Read the model definition and answer for the solid it produces. Units are mm, in the model's axes. Face numbers are marked on the shaded views. A direction names the side the tool comes from. Coordinates: 2 decimals unless noted, no trailing zeros. Order: outer loops, then holes, each group sorted by start corner. A loop starts at its lowest first (then second) coordinate and runs counter-clockwise, first axis right, second up. Notation, with made-up numbers: M 14,-8.5 L 56,-8.5 A9 cw 56,4.5 Z; hole C -22,74.25 d4. An arc over 180 degrees is marked long. Put each result on its own line as item: value.
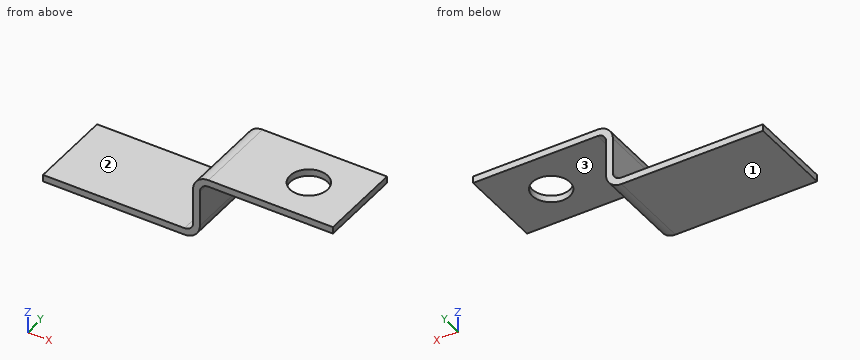
from build123d import *

# Parameters (mm, degrees)
SKETCH1_W           = 34
SKETCH1_H           = 10
BOSS_EXTRUDE1_DEPTH = 7.8
SKETCH2_W           = 15.6
SKETCH2_H           = 7
CUT_EXTRUDE1_DEPTH  = 63.432123894
SKETCH3_W           = 17.6
SKETCH3_H           = 7
CUT_EXTRUDE2_DEPTH  = 63.432123894
HOLE1_D             = 4.4
HOLE1_DEPTH         = 7.8
FILLET1_R           = 1
FILLET2_R           = 1
FILLET3_R           = 1.8
FILLET4_R           = 1.8


with BuildPart() as part:
    # Sketch1 → Boss-Extrude1 (new body)
    with BuildSketch(Plane.XY.offset(4.484761641)):
        with Locations((-44.46264725, 0)):
            Rectangle(SKETCH1_W, SKETCH1_H)
    extrude(amount=-BOSS_EXTRUDE1_DEPTH)

    # Sketch2 → Cut-Extrude1 (cut, through all)
    with BuildSketch(Plane(origin=(0, 5, 0), x_dir=(-1, 0, 0), z_dir=(0, 1, 0))):
        with Locations((35.26264725, 0.184761641)):
            Rectangle(SKETCH2_W, SKETCH2_H)
    extrude(amount=-CUT_EXTRUDE1_DEPTH, mode=Mode.SUBTRACT)

    # Sketch3 → Cut-Extrude2 (cut, through all)
    with BuildSketch(Plane(origin=(0, 5, 0), x_dir=(-1, 0, 0), z_dir=(0, 1, 0))):
        with Locations((52.66264725, 0.984761641)):
            Rectangle(SKETCH3_W, SKETCH3_H)
    extrude(amount=-CUT_EXTRUDE2_DEPTH, mode=Mode.SUBTRACT)

    # Hole1
    with Locations(Plane.XY.offset(4.484761641)):
        with Locations((-33.46264725, 0)):
            Hole(HOLE1_D / 2, depth=HOLE1_DEPTH)

    # Fillet1
    fillet1_edges = [part.edges().sort_by_distance(p)[0] for p in [
        (-43.06264725, 0, 3.684761641),
    ]]
    fillet(fillet1_edges, radius=FILLET1_R)

    # Fillet2
    fillet2_edges = [part.edges().sort_by_distance(p)[0] for p in [
        (-43.86264725, 0, -2.515238359),
    ]]
    fillet(fillet2_edges, radius=FILLET2_R)

    # Fillet3
    fillet3_edges = [part.edges().sort_by_distance(p)[0] for p in [
        (-43.06264725, 0, -3.315238359),
    ]]
    fillet(fillet3_edges, radius=FILLET3_R)

    # Fillet4
    fillet4_edges = [part.edges().sort_by_distance(p)[0] for p in [
        (-43.86264725, 0, 4.484761641),
    ]]
    fillet(fillet4_edges, radius=FILLET4_R)


solid = part.part
Q1. A tool of negligible diameter and unlimited length cuts with its end or side. For the marked faces 1, 2 and 3, from which of +Z, -Z, +X, -X, +Y, -Y can it reach the whole face along a straight path? Write none if from no direction.
Answers below:
face 1: -Z, +X, -X, +Y, -Y
face 2: +Z, -X, +Y, -Y
face 3: -Z, +X, +Y, -Y
Q2. Find section B-B on x = -35. Write down the section's boundary in (y, z), plus the area to 3 significant figures.
Answers below:
outline: M -5,3.68 L -1.57,3.68 L -1.57,4.48 L -5,4.48 Z; M 1.57,3.68 L 5,3.68 L 5,4.48 L 1.57,4.48 Z
area: 5.48 mm^2
Q3. Find section A-A on y = -1.75. Write down the section's boundary in (x, z), plus the area to 3 significant figures.
Answers below:
outline: M -61.46,-3.32 L -44.86,-3.32 A1.8 ccw -43.06,-1.52 L -43.06,2.68 A1 cw -42.06,3.68 L -34.8,3.68 L -34.8,4.48 L -42.06,4.48 A1.8 ccw -43.86,2.68 L -43.86,-1.52 A1 cw -44.86,-2.52 L -61.46,-2.52 Z; M -32.13,3.68 L -27.46,3.68 L -27.46,4.48 L -32.13,4.48 Z
area: 29.7 mm^2
Q4. Find section C-C on y = 2.5. Write down the section's boundary in (x, z), plus the area to 3 significant figures.
Answers below:
outline: M -61.46,-3.32 L -44.86,-3.32 A1.8 ccw -43.06,-1.52 L -43.06,2.68 A1 cw -42.06,3.68 L -27.46,3.68 L -27.46,4.48 L -42.06,4.48 A1.8 ccw -43.86,2.68 L -43.86,-1.52 A1 cw -44.86,-2.52 L -61.46,-2.52 Z
area: 31.8 mm^2
Q5. Given pin 1 (4 mm diameter, centred on x = -53.5, y = -2, fed in from +Z); pin 2 (2 mm diameter, centred on x = -41, y = 3, fed in from -Z); pin 3 (3 mm diameter, centred on x = -44, y = 3.5, fed in from +Z); pin 4 (5.5 mm diameter, centred on x = -33.46, y = 0, fed in from +Z), each flat-ended and moving along its own axis, determine where each tip first touches the part or whether it passes through.
Answers below:
pin 1: stops at z = -2.52
pin 2: stops at z = 3.68
pin 3: stops at z = 4.43
pin 4: stops at z = 4.48
Q6. Find section D-D on x = -55. Write down the section's boundary in (y, z).
Answers below:
outline: M -5,-3.32 L 5,-3.32 L 5,-2.52 L -5,-2.52 Z
Q7. Consider line 1 along Z through (x, y) = (-54, 3.5); line 2 along Z through (x, y) = (-39, 3.5); line 3 along X through (y, z) = (-0.5, 1.5). Determine where each line is inside the solid, lowest interval first.
Answers below:
line 1: z = -3.32 to -2.52
line 2: z = 3.68 to 4.48
line 3: x = -43.86 to -43.06
